Design review of the part built by this model. Coordinates are the model's own, in mm. A direction names the side the tool comes from. Give positions to 0.01 mm unless a question says otherwise; leave off trailing zeros. Write each loop counter-clockwise with the first axis right and the second up, starting at its lowest first coordinate (ties: lowest second). Pieces come first, ordered by that corner, then holes.
```python
from build123d import *

# Parameters (mm, degrees)
F0_W     = 27.1828
F0_H     = 76
F0_W_2   = 14.4828
F0_H_2   = 63.3
F1_DEPTH = 5.842
F2_R     = 0.198438
F3_DEPTH = 5.843


with BuildPart() as f1:
    # F0 (on Front) → F1 (new body)
    with BuildSketch(Plane.XZ):
        Rectangle(F0_W, F0_H)
        Rectangle(F0_W_2, F0_H_2, mode=Mode.SUBTRACT)
    extrude(amount=F1_DEPTH)

    # F2 (on face) → F3 (cut, through all)
    with BuildSketch(Plane.XZ.offset(5.842)):
        with Locations((-7.2414, 31.65)):
            Circle(F2_R)
        with Locations((7.2414, 31.65)):
            Circle(F2_R)
        with Locations((-7.2414, -31.65)):
            Circle(F2_R)
        with Locations((7.2414, -31.65)):
            Circle(F2_R)
    extrude(amount=-F3_DEPTH, mode=Mode.SUBTRACT)


solid = f1.part
```
(1) Consider section C-C, the plane x = -2. Give the boundary of the cut face in (y, z).
Resolved:
outline: (-5.84, -38) - (0, -38) - (0, -31.65) - (-5.84, -31.65) - close; (-5.84, 31.65) - (0, 31.65) - (0, 38) - (-5.84, 38) - close
(2) To check wall thickness, follow L1, parallel to Z at x = 5, y = -1.4; L2, parallel to X at y = -3.75, z = 9. State the ranges of each line that lie inside material, in increasing order.
Resolved:
L1: z = -38 to -31.65, 31.65 to 38
L2: x = -13.59 to -7.24, 7.24 to 13.59
(3) Consider section B-B, the plane z = 14. Give the boundary of the cut face in (x, y).
Resolved:
outline: (-13.59, -5.84) - (-7.24, -5.84) - (-7.24, 0) - (-13.59, 0) - close; (7.24, -5.84) - (13.59, -5.84) - (13.59, 0) - (7.24, 0) - close
(4) Mouldability with a two-part tool opening along X and no side actions: class faces 3 (the face through (0, -3, -31.65)), 4 (the face through (-7.241, -3, 0)), 5 (the face through (-13.591, -3, -1)), 6 (the face through (13.591, -3, -1)) as pulls with the +X half, pulls with the -X half, needs draft (parallel to the pull), parting line crosses it, or undercut.
Resolved:
face 3: undercut
face 4: undercut
face 5: pulls with the -X half
face 6: pulls with the +X half
(5) Consider section A-A, the plane y = -4.35. Give the boundary of the cut face in (x, z).
Resolved:
outline: (-13.59, -38) - (13.59, -38) - (13.59, 38) - (-13.59, 38) - close; hole (-7.24, -31.45) arc R0.2 ccw (long way) to (-7.04, -31.65) - (7.04, -31.65) arc R0.2 ccw (long way) to (7.24, -31.45) - (7.24, 31.45) arc R0.2 ccw (long way) to (7.04, 31.65) - (-7.04, 31.65) arc R0.2 ccw (long way) to (-7.24, 31.45) - close
(6) Tool access review of faces 1 (the face through (0, -3, 31.65)), 2 (the face through (0, -3, -38)): name each direction out of +Z, -Z, +X, -X, +Y, -Y from which nothing blocks a thin tool from reaching the whole face with its end or side.
Resolved:
face 1: +Y, -Y
face 2: -Z, +X, -X, +Y, -Y
